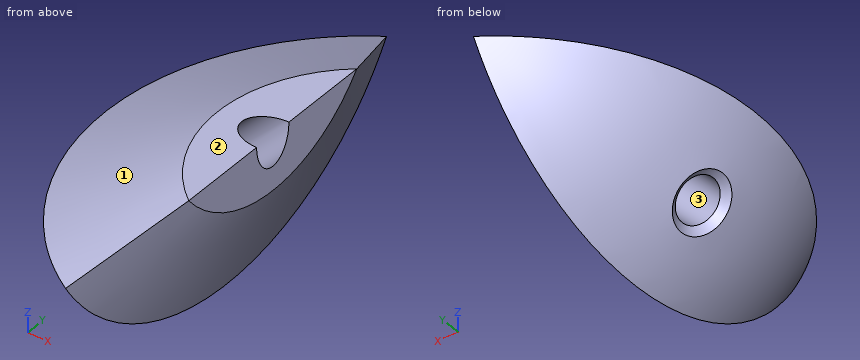
from build123d import *
from OCP.BRepAlgoAPI import BRepAlgoAPI_Cut
from OCP.TopTools import TopTools_ListOfShape

# Parameters (mm, degrees)
CUT_EXTRUDE_1_DEPTH      = 59.108987417
CUT_EXTRUDE_1_DEPTH_BACK = 59.108987417
CUT_EXTRUDE_2_DEPTH      = 59.108987417
CUT_EXTRUDE_2_DEPTH_BACK = 59.108987417
SKETCH_12_W              = 3
SKETCH_12_H              = 50.62024983


with BuildPart() as part:
    # 草图3 → 旋转1 (revolve)
    with BuildSketch(Plane(origin=(0, 0, 0), x_dir=(0, 0, -1), z_dir=(1, 0, 0))):
        with BuildLine():
            Line((0, 40), (0, -40))
            ThreePointArc((0, -40), (40, 0), (0, 40))
        make_face()
    revolve(axis=Axis((0, 40, 0), (0, -1, 0)))

    # 草图4 → 切除-旋转3 (revolve, cut)
    with BuildSketch(Plane.XY, mode=Mode.PRIVATE) as cut_revolve_3_sk:
        Polygon((-25, 50), (25, 50), (12.5, 20), (-12.5, 20), align=None)
    revolve(cut_revolve_3_sk.sketch.rotate(Axis((-55.247864245, 0, 0), (1, 0, 0)), 90), axis=Axis((-55.247864245, 0, 0), (1, 0, 0)), mode=Mode.SUBTRACT)


with BuildPart() as cut_revolve_4_tool:
    # 草图5 → 切除-旋转4 (revolve)
    with BuildSketch(Plane(origin=(0, 0, 0), x_dir=(1, 0, 0), z_dir=(0, 1, 0))):
        Polygon((-50, 25), (-50, -25), (-20, -12.5), (-20, 12.5), align=None)
    revolve(axis=Axis((0, 0, -44.002313129), (0, 0, 1)))


with BuildPart() as part_1:
    add(part.part)

    # 切除-旋转4: cut by cut_revolve_4_tool, with a tolerance
    cut_revolve_4_stock = TopTools_ListOfShape()
    cut_revolve_4_stock.Append(part_1.part.wrapped)
    cut_revolve_4_tools = TopTools_ListOfShape()
    cut_revolve_4_tools.Append(cut_revolve_4_tool.part.wrapped)
    cut_revolve_4_cut = BRepAlgoAPI_Cut()
    cut_revolve_4_cut.SetArguments(cut_revolve_4_stock)
    cut_revolve_4_cut.SetTools(cut_revolve_4_tools)
    cut_revolve_4_cut.SetFuzzyValue(0.00001)
    cut_revolve_4_cut.Build()
    add(Compound.cast(cut_revolve_4_cut.Shape()).solids(), mode=Mode.REPLACE)

    # 草图6 → 切除-拉伸1 (cut, two sides: drawn at the far end of the back side and taken through both)
    with BuildSketch(Plane(origin=(0, 0, 0), x_dir=(1, 0, 0), z_dir=(0, 1, 0)).offset(-CUT_EXTRUDE_1_DEPTH_BACK)):
        Polygon((-20, 12.5), (37.556288363, 12.5), (37.556288363, -29.25786606), (31.486585193, -38.646938151), (-34.426597666, -38.077903479), (-43.720830645, -12.186825895), align=None)
    extrude(amount=CUT_EXTRUDE_1_DEPTH + CUT_EXTRUDE_1_DEPTH_BACK, mode=Mode.SUBTRACT)

    # 草图7 → 切除-拉伸2 (cut, two sides: drawn at the far end of the back side and taken through both)
    with BuildSketch(Plane(origin=(0, 0, 0), x_dir=(1, 0, 0), z_dir=(0, 1, 0)).offset(-CUT_EXTRUDE_2_DEPTH_BACK)):
        Polygon((-12.5, 20), (-10.113298037, 50.085656358), (42.871589505, 47.227550391), (40.63466159, 5.758348279), (-0.879417221, -1.726674889), (-12.5, 12.5), align=None)
    extrude(amount=CUT_EXTRUDE_2_DEPTH + CUT_EXTRUDE_2_DEPTH_BACK, mode=Mode.SUBTRACT)

    # 草图12 → 切除-旋转7 (revolve, cut)
    with BuildSketch(Plane(origin=(0, 0, 0), x_dir=(0, 1, 0), z_dir=(0.7071067811865464, 0, -0.7071067811865488)), mode=Mode.PRIVATE) as cut_revolve_7_sk:
        with Locations((1.5, -25.310124915)):
            Rectangle(SKETCH_12_W, SKETCH_12_H)
    revolve(cut_revolve_7_sk.sketch.rotate(Axis((0, 0, 0), (-0.7071067811865488, 0, -0.7071067811865464)), 90), axis=Axis((0, 0, 0), (-0.7071067811865488, 0, -0.7071067811865464)), mode=Mode.SUBTRACT)

    # 倒角1
    # the kernel refuses this chamfer: 1, 0.93267614 mm, written as the material it takes off along each edge
    with BuildSketch(Plane(origin=(-28.204609567, 1e-09, -28.204609538), x_dir=(0.7071067811865464, -3.5887694896846076e-10, -0.7071067811865487), z_dir=(2.537647002539835e-10, 1.0, -2.537639482002908e-10))) as chamfer_1_piece_1:
        with BuildLine():
            Line((3.984104251, -0.086249492), (2.999999979, -0.932676176))
            Line((2.999999979, -0.932676176), (3.000000021, 0))
            ThreePointArc((3.000000021, 0), (3.506227368, -0.041308053), (3.984104251, -0.086249492))
        make_face()
    revolve(axis=Axis((-28.204609567, 1e-09, -28.204609538), (-0.7071067811865486, 0, -0.7071067811865465)), mode=Mode.SUBTRACT)


solid = part_1.part
Build history of the part. All positions in model axes, mm. Face numbers are marked on the shaded views. Round coordinates to 2 decimals unless told otherwise and drop trailing zeros. Use CSV: the item, a comma, the result in double quotes. Start each with the question number.
(1) Mould opens along X. For the marked faces 1, 2 and 3 say: +X half, -X half, draft (parallel to the pull), parting line (faces both ways), or undercut.
(2) Drill centre lines: probe 1 along Y at (x, z) = (-21.75, -25.5); probe 2 along Y at (x, z) = (-24.5, -24.75); probe 3 along Z at (x, y) = (-20.5, 0.5). Where is each one in solid material? Low to high.
(3) Flat gauge pins, fed straight in: P1, Ø1.5, axis at y = 4.5, z = -22, coming from the +X side; P2, Ø5, axis at x = -27.5, y = -13, coming from the -Z side; P3, Ø5, axis at y = -20.5, z = -30, coming from the -X side. Where does each tip first touch, or does it go through?
Findings:
1,face 1,"-X half"
1,face 2,"draft"
1,face 3,"undercut"
2,probe 1,"y = -21.83 to -1.4, 1.4 to 21.83"
2,probe 2,"y = -19.68 to -2.99, 2.99 to 19.68"
2,probe 3,"z = -34.34 to -24.68, -16.32 to -12.71"
3,P1,"stops at x = -13.21"
3,P2,"stops at z = -28.65"
3,P3,"stops at x = -21.33"
